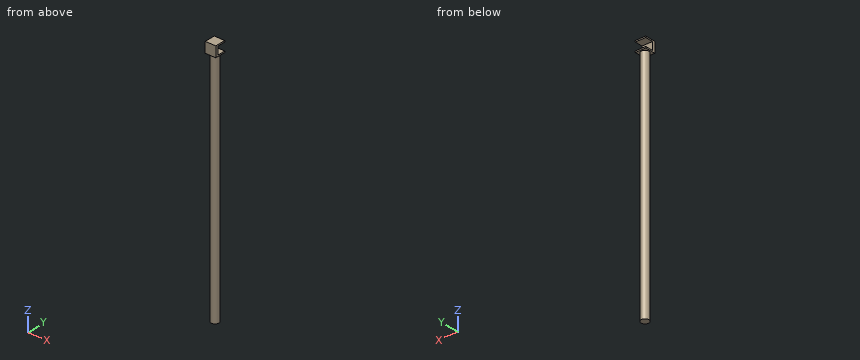
from build123d import *

# Parameters (mm, degrees)
BOSS_EXTRUDE1_DEPTH = 10
SKETCH4_R           = 7.5
BOSS_EXTRUDE2_DEPTH = 450


with BuildPart() as part:
    # Sketch2 → Boss-Extrude1 (new, symmetric)
    with BuildSketch(Plane(origin=(0, 0, 0), x_dir=(0, 0, -1), z_dir=(1, 0, 0))):
        Polygon((7.5, 7.5), (10, 7.5), (10, -12.5), (-10, -12.5), (-10, 7.5), (-7.5, 7.5), (-7.5, -7.5), (7.5, -7.5), align=None)
    extrude(amount=BOSS_EXTRUDE1_DEPTH, both=True)

    # Sketch4 → Boss-Extrude2 (add)
    with BuildSketch(Plane(origin=(0, 0, -10), x_dir=(-1, 0, 0), z_dir=(0, 0, -1))):
        with Locations(Location((0, -2.5, 0), (0, 0, 90))):
            Circle(SKETCH4_R)
    extrude(amount=BOSS_EXTRUDE2_DEPTH)


solid = part.part
Geometry check sheet. Reference: the model listing, model coordinates, mm. Coordinates: 2 decimals unless noted, no trailing zeros. Order: outer loops, then holes, each group sorted by start corner. A loop starts at its lowest first (then second) coordinate and runs counter-clockwise, first axis right, second up. Notation, with made-up numbers: (28, -27) - (34, -27) arc R13 cw to (34, -8) - close; hole circle Ø4 at (58.25, 76). An arc over 180 degrees is marked (long way). Answer in a Markdown table with one row per item. Add a question column.
1) Gauge pin test, flat ends, axial feed: P1, Ø6, axis at y = -3, z = -101, coming from the -X side; P2, Ø4.5, axis at x = 4, z = -1, coming from the +Y side; P3, Ø8, axis at x = -4.5, z = -389.5, coming from the -Y side. Record the tip position at first contact, or that the pin passes through.
2) Cross-section at B-B, the plane x = 0. Record the cut outline in (y, z), then the cut area to 4 significant figures.
3) Cross-section at C-C, the plane z = -312.5. Record the cut outline in (x, y), then the cut area to 3 significant figures.
4) Cross-section at A-A, the plane y = -2.5. Record the cut outline in (x, z), then the cut area to 3 significant figures.
5) Material ranges on line 1 along Z through (x, y) = (7.75, -0.75); line 2 along Z through (x, y) = (-5, -1); line 3 along Z through (x, y) = (-6.25, -11.5), recorded low to high. Write a range as [from, to].
Check result:
| question | item | result |
|---|---|---|
| 1 | P1 | stops at x = -7.5 |
| 1 | P2 | stops at y = -7.5 |
| 1 | P3 | stops at y = -9.98 |
| 2 | outline | (-12.5, -10) - (-10, -10) - (-10, -460) - (5, -460) - (5, -10) - (7.5, -10) - (7.5, -7.5) - (-7.5, -7.5) - (-7.5, 7.5) - (7.5, 7.5) - (7.5, 10) - (-12.5, 10) - close |
| 2 | area | 6,925 mm² |
| 3 | outline | circle Ø15 at (0, -2.5) |
| 3 | area | 177 mm² |
| 4 | outline | (-10, -10) - (-7.5, -10) - (-7.5, -460) - (7.5, -460) - (7.5, -10) - (10, -10) - (10, -7.5) - (-10, -7.5) - close; (-10, 7.5) - (10, 7.5) - (10, 10) - (-10, 10) - close |
| 4 | area | 6,850 mm² |
| 5 | line 1 | z = [-10, -7.5], [7.5, 10] |
| 5 | line 2 | z = [-460, -7.5], [7.5, 10] |
| 5 | line 3 | z = [-10, 10] |
